Geometry: see drawing. Coordinates: mm, zero at the bounding-box minimum. A direction names the side the tool comes from. Coordinates: 2 decimals unless noted, no trailing zeros. Write each loop counter-clockwise with the first axis right and the second up, starting at its lowest first coordinate (ties: lowest second). Pieces come first, ordered by that corner, then holes. Notation, with made-up numbers: (89, 12.25) - (108, 12.25) arc R29 cw to (108, 40.25) - close; hole circle Ø8 at (11.5, 6.25). An arc over 180 degrees is marked (long way). One line per question, with ' | ' between items. Start each with the question number.
Q1. Cut plane A-A, the plane x = 8.1. Return loops of the section in (y, z).
Q2. Cut plane C-C, the plane y = 19.5. Return loops of the section in (x, z), plus the area to 3 significant figures.
Q3. Contact query for flat-ended pins moving along their axis: P1, Ø14, axis at y = 8, z = 15, coming from the -X side; P2, Ø3, axis at x = 8, z = 14, coming from the +Y side; P3, Ø0.6, axis at x = 8, z = 30.5, coming from the -Y side; P4, Ø7, axis at x = 8.1, z = 21.9, coming from the +Y side. Output: stop coordinate, or through.
Q4. Line query: line 1 (Z direction, x = 8, y = 1.5); line 2 (Z direction, x = 4.75, y = 16.75); line 3 (X direction, y = 4.5, z = 2.65). Output: solid intervals per line, ascending.
Q5. Cut plane B-B, the plane z = 21.9. Return loops of the section in (x, y).
Q6. Access query for the marked faces 1 and 2. Directions: +Z, -Z, +X, -X, +Y, -Y. A direction counts if a zero-diameter tool reaches every point of the face in a straight line with its end or side. Return the directions, or none.
Q7. Draft query along Z for the marked faces 3, 4, 5 and 6. Return one class per face: +Z half, -Z half, draft (parallel to the pull), parting line (faces both ways), or undercut.
Q8. Cut plane D-D, the plane z = 30.15. Return loops of the section in (x, y).
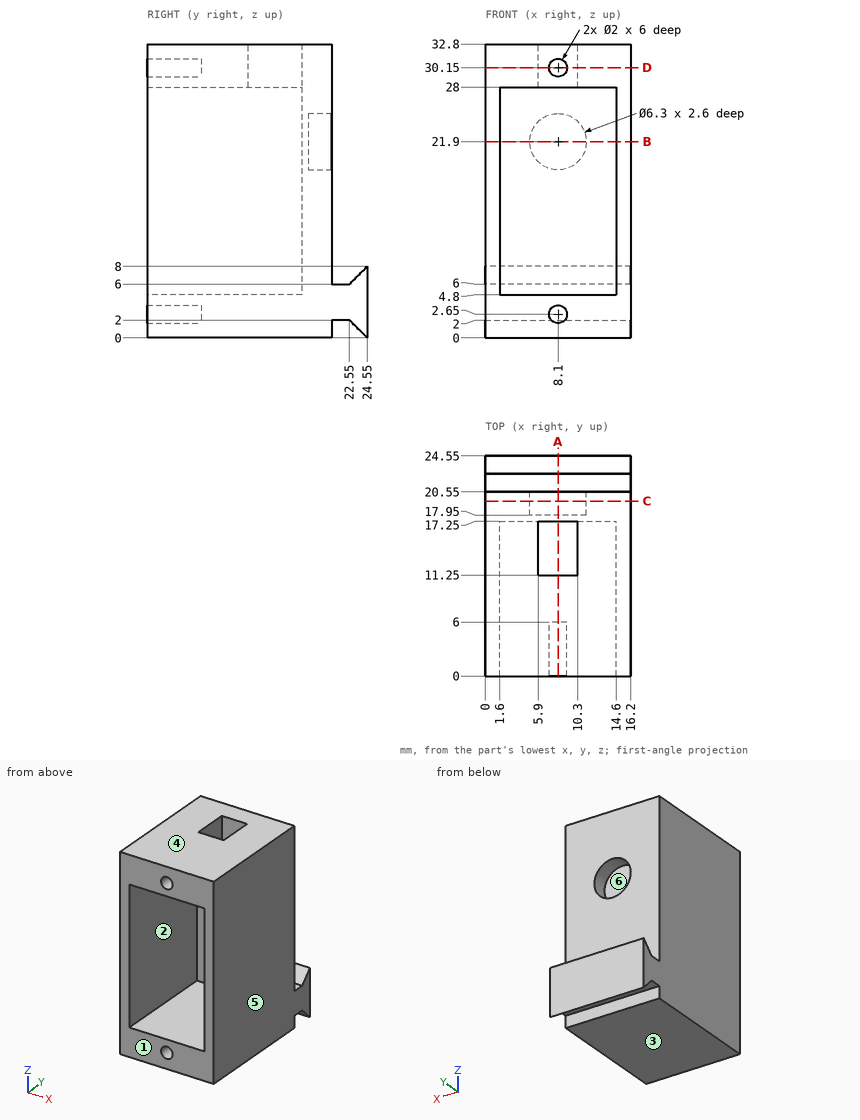
Reply:
1) outline: (0, 0) - (20.55, 0) - (20.55, 2) - (22.55, 2) - (24.55, 0) - (24.55, 8) - (22.55, 6) - (20.55, 6) - (20.55, 18.75) - (17.95, 18.75) - (17.95, 25.05) - (20.55, 25.05) - (20.55, 32.8) - (17.25, 32.8) - (17.25, 4.8) - (0, 4.8) - (0, 3.65) - (6, 3.65) - (6, 1.65) - (0, 1.65) - close; (0, 28) - (11.25, 28) - (11.25, 32.8) - (0, 32.8) - (0, 31.15) - (6, 31.15) - (6, 29.15) - (0, 29.15) - close
2) outline: (0, 0) - (16.2, 0) - (16.2, 32.8) - (0, 32.8) - close; hole circle Ø6.3 at (8.1, 21.9) | area: 500 mm^2
3) P1: stops at x = 0 | P2: stops at y = 20.55 | P3: stops at y = 6 | P4: stops at y = 20.55
4) line 1: z = 0 to 1.66, 3.64 to 4.8, 28 to 29.16, 31.14 to 32.8 | line 2: z = 0 to 4.8, 28 to 32.8 | line 3: x = 0 to 7.1, 9.1 to 16.2
5) outline: (0, 0) - (1.6, 0) - (1.6, 17.25) - (14.6, 17.25) - (14.6, 0) - (16.2, 0) - (16.2, 20.55) - (11.25, 20.55) - (11.25, 17.95) - (4.95, 17.95) - (4.95, 20.55) - (0, 20.55) - close
6) face 1: +Z, -Z, +X, -X, -Y | face 2: -Y
7) face 3: -Z half | face 4: +Z half | face 5: draft | face 6: undercut
8) outline: (0, 0) - (7.1, 0) - (7.1, 6) - (9.1, 6) - (9.1, 0) - (16.2, 0) - (16.2, 20.55) - (0, 20.55) - close; hole (5.9, 11.25) - (10.3, 11.25) - (10.3, 17.25) - (5.9, 17.25) - close
